Design review of the part built by this model. Coordinates are the model's own, in mm. A direction names the side the tool comes from. Give positions to 0.01 mm unless a question says otherwise; leave off trailing zeros. Loops run counter-clockwise (first coordinate to the right, second up) from the corner with the lowest first, then second, coordinate; pieces in that order, holes last.
Autodesk Fusion 360 part; units mm, degrees
sketch "Sketch1" plane through (0, 0, 0) normal (0, 0, 1) x (1, 0, 0)
  line L0 (0, 0) -> (-30, 0)
  line L1 (-30, 0) -> (-30, 30)
  line L2 (-30, 30) -> (0, 30)
  line L3 (0, 30) -> (0, 0)
  dimension "d1" = 30
  dimension "d2" = 30
extrude "Extrude1" add sketch "Sketch1" along normal blind 30
sketch "Sketch2" plane through (0, 0, 30) normal (0, 0, 1) x (-1, 0, 0)
  line L0 (0, -30) -> (30, -30)
  line L1 (30, -30) -> (30, 0)
  line L2 (30, 0) -> (0, 0)
  line L3 (0, 0) -> (0, -30)
  line L4 (30, 0) -> (25.5, 0)
  line L5 (25.5, 0) -> (25.5, -2)
  line L6 (25.5, -2) -> (30, -2)
  line L7 (30, -2) -> (30, 0)
  line L8 (25.5, -2) -> (4.5, -2)
  line L9 (4.5, -2) -> (4.5, -9)
  line L10 (4.5, -9) -> (25.5, -9)
  line L11 (25.5, -9) -> (25.5, -2)
  dimension "d5" = 4.5
  dimension "d6" = 2
  dimension "d7" = 21
  dimension "d8" = 7
extrude "Extrude2" cut sketch "Sketch2" against normal blind 25 contours L8 L9 L10 L11
sketch "Sketch3" plane through (0, 0, 0) normal (0, -1, 0) x (1, 0, 0)
  line L0 (-30, 0) -> (0, 0)
  line L1 (0, 0) -> (0, 30)
  line L2 (0, 30) -> (-30, 30)
  line L3 (-30, 30) -> (-30, 0)
  line L4 (-6, 6) -> (-24, 6)
  line L5 (-24, 6) -> (-24, 24)
  line L6 (-24, 24) -> (-6, 24)
  line L7 (-6, 24) -> (-6, 6)
  line L8 (-6, 6) -> (-24, 24) construction
  line L9 (-24, 6) -> (-6, 24) construction
  point P0 (-15, 15)
  dimension "d11" = 18
  dimension "d12" = 18
extrude "Extrude3" cut sketch "Sketch3" against normal blind 2 contours L4 L5 L6 L7
sketch "Sketch4" plane through (0, 0, 0) normal (1, 0, 0) x (0, 1, 0)
  line L0 (0, 0) -> (30, 0)
  line L1 (30, 0) -> (30, 30)
  line L2 (30, 30) -> (0, 30)
  line L3 (0, 30) -> (0, 0)
  line L4 (0, 0) -> (2, 0)
  line L5 (2, 0) -> (2, 30)
  line L6 (2, 30) -> (0, 30)
  line L7 (0, 30) -> (0, 0)
  dimension "d15" = 2
  dimension "d16" = 30
extrude "Extrude4" add sketch "Sketch4" along normal blind 2 contours L0 L2 L3 L4 L5 L6 L7
sketch "Sketch5" plane through (-30, 0, 0) normal (-1, 0, 0) x (0, -1, 0)
  line L0 (-30, 0) -> (0, 0)
  line L1 (0, 0) -> (0, 30)
  line L2 (0, 30) -> (-30, 30)
  line L3 (-30, 30) -> (-30, 0)
  line L4 (0, 0) -> (-2, 0)
  line L5 (-2, 0) -> (-2, 30)
  line L6 (-2, 30) -> (0, 30)
  line L7 (0, 30) -> (0, 0)
  dimension "d19" = 2
  dimension "d20" = 30
extrude "Extrude5" add sketch "Sketch5" along normal blind 2 contours L0 L1 L2 L4 L5 L6 L7
sketch "Sketch6" plane through (0, 0, 5) normal (0, 0, 1) x (-1, 0, 0)
  line L0 (25.5, -9) -> (25.5, -2)
  line L1 (25.5, -2) -> (4.5, -2)
  line L2 (4.5, -2) -> (4.5, -9)
  line L3 (4.5, -9) -> (25.5, -9)
  circle A0 centre (6, -5) radius 1
  dimension "d23" = 2
extrude "Extrude6" cut sketch "Sketch6" against normal blind 5 contours A0
sketch "Sketch7" plane through (0, 0, 0) normal (0, -1, 0) x (1, 0, 0)
  line L0 (-24, 6) -> (-24, 24)
  line L1 (-24, 24) -> (-6, 24)
  line L2 (-6, 24) -> (-6, 6)
  line L3 (-6, 6) -> (-24, 6)
  line L4 (-32, 0) -> (2, 0)
  line L5 (2, 0) -> (2, 30)
  line L6 (2, 30) -> (-32, 30)
  line L7 (-32, 30) -> (-32, 0)
  line L8 (-6, 6) -> (-24, 6)
  line L9 (-24, 6) -> (-24, 24)
  line L10 (-24, 24) -> (-6, 24)
  line L11 (-6, 24) -> (-6, 6)
extrude "Extrude7" cut sketch "Sketch7" against normal blind 28 contours L0 L1 L2 L3 L8 L9 L10 L11
fillet "Fillet1" radius 10 1 edges at (-15, 30, 30)
sketch "Sketch8" plane through (0, 0, 6) normal (0, 0, 1) x (-1, 0, 0)
  line L0 (24, -9) -> (6, -9)
  line L1 (6, -9) -> (6, -28)
  line L2 (6, -28) -> (24, -28)
  line L3 (24, -28) -> (24, -9)
  line L4 (24, -28) -> (6, -28)
  line L5 (6, -28) -> (6, -9)
  line L6 (6, -9) -> (24, -9)
  line L7 (24, -9) -> (24, -28)
sketch "Sketch9" plane through (0, 0, 6) normal (0, 0, 1) x (-1, 0, 0)
  line L0 (6, -9) -> (8, -9)
  line L1 (8, -9) -> (8, -11)
  line L2 (8, -11) -> (6, -11)
  line L3 (6, -11) -> (6, -9)
  line L4 (6, -11) -> (24, -11)
  line L5 (24, -11) -> (24, -28)
  line L6 (24, -28) -> (6, -28)
  line L7 (6, -28) -> (6, -11)
  point P0 (6, -9)
  point P1 (24, -28)
  dimension "d30" = 2
  dimension "d31" = 2
extrude "Extrude8" cut sketch "Sketch9" against normal blind 10 contours L2 L4 L5 L6 L7
extrude "Extrude9" cut 1 faces at (-29.3333, 0, 18) along direction (0, 1, 0) blind 0.2
sketch "Sketch10" plane through (0, 0, 0) normal (0, 0, -1) x (1, 0, 0)
  line L0 (2, -0.2) -> (-32, -0.2)
  line L1 (-32, -0.2) -> (-32, -2)
  line L2 (-32, -2) -> (-30, -2)
  line L3 (-30, -2) -> (-30, -30)
  line L4 (-30, -30) -> (0, -30)
  line L5 (0, -30) -> (0, -2)
  line L6 (0, -2) -> (2, -2)
  line L7 (2, -2) -> (2, -0.2)
  circle A0 centre (-6, -5) radius 1
  line L8 (-24, -28) -> (-24, -11)
  line L9 (-24, -11) -> (-6, -11)
  line L10 (-6, -11) -> (-6, -28)
  line L11 (-6, -28) -> (-24, -28)
extrude "Extrude10" add sketch "Sketch10" against normal blind 5 contours A0
extrude "Extrude11" cut 1 faces at (-11.5, 6.6667, 5) along direction (0, 0, -1) blind 1
sketch "Sketch11" plane through (0, 0, 4) normal (0, 0, 1) x (-1, 0, 0)
  line L0 (25.5, -9) -> (25.5, -2)
  line L1 (25.5, -2) -> (4.5, -2)
  line L2 (4.5, -2) -> (4.5, -9)
  line L3 (4.5, -9) -> (25.5, -9)
  circle A0 centre (8.1497, -5.5) radius 2
  dimension "d40" = 4
extrude "Extrude12" cut sketch "Sketch11" against normal blind 4 contours A0
extrude "Extrude13" cut 1 faces at (2, 0.8, 20) along direction (-1, 0, 0) blind 0.2
extrude "Extrude14" cut 1 faces at (-32, 1.4, 20) along direction (1, 0, 0) blind 0.2
extrude "Extrude15" cut 1 faces at (1.8, 0.8, 20) along direction (-1, 0, 0) blind 0.1
extrude "Extrude16" cut 1 faces at (-29.2, 0.2, 18) along direction (0, 1, 0) blind 0.2
extrude "Extrude17" cut 1 faces at (-31.8, 1.4667, 20) along direction (1, 0, 0) blind 0.1
Q1. Insertion check: pin 1 (5 mm diameter, centred on y = 8.5, z = 16, fed in from -X); pin 2 (2 mm diameter, centred on x = -8, z = 24.5, fed in from +Y); pin 3 (8 mm diameter, centred on x = -19.5, y = 23.5, fed in from -Z); pin 4 (3.5 mm diameter, centred on x = -8.15, y = 5.5, fed in from -Z). Each pin has a flat end and moves straight along its axis. Give the tip position at first contact, or say it passes through.
Results:
pin 1: stops at x = -30
pin 2: stops at y = 29.37
pin 3: stops at z = 24
pin 4: passes through
Q2. Take a section at A-A (y = 5.5). Give the boundary of the cut face in (x, z), plus the area to 3 significant figures.
Results:
outline: (-30, 0) - (-10.15, 0) - (-10.15, 4) - (-25.5, 4) - (-25.5, 30) - (-30, 30) - close; (-6.15, 0) - (0, 0) - (0, 30) - (-4.5, 30) - (-4.5, 4) - (-6.15, 4) - close
area: 338 mm2
Q3. Take a section at B-B (z = 3.25). Give the boundary of the cut face in (x, y), plus the area to 3 significant figures.
Results:
outline: (-31.7, 0.4) - (1.7, 0.4) - (1.7, 2) - (0, 2) - (0, 30) - (-30, 30) - (-30, 2) - (-31.7, 2) - close; hole (-24, 11) - (-6, 11) - (-6, 28) - (-24, 28) - close; hole circle Ø4 at (-8.15, 5.5)
area: 575 mm2
Q4. Take a section at D-D (y = 18.25). Give the boundary of the cut face in (x, z), plus the area to 3 significant figures.
Results:
outline: (-30, 0) - (-24, 0) - (-24, 24) - (-6, 24) - (-6, 0) - (0, 0) - (0, 30) - (-30, 30) - close
area: 468 mm2
Q5. Tool access review of faces 4 (the face through (-25.5, 6, 17)), 5 (the face through (-15, 11, 3)), 6 (the face through (-15, 10, 6)): name each direction out of +Z, -Z, +X, -X, +Y, -Y from which nothing blocks a thin tool from reaching the whole face with its end or side.
Results:
face 4: +Z
face 5: -Z
face 6: -Y
Q6. Draft analysis for pull direction X (two halves, no side actions). For faces 1 (the face through (-9.997, 6.266, 2.028)), 2 (the face through (1, 2, 15)), 3 (the face through (0, 16, 15)), state which applies: pulls with the +X half, pulls with the -X half, needs draft (parallel to the pull), parting line crosses it, or undercut.
Results:
face 1: undercut
face 2: needs draft
face 3: pulls with the +X half
Q7. Wall thickness on line 1 (X direction, y = 22, z = 9.5); line 2 (Y direction, x = -5, z = 7); line 3 (X direction, y = 5.5, z = 1.5): over which ranges is each line inside the solid? List them lowest first.
Results:
line 1: x = -30 to -24, -6 to 0
line 2: y = 0.4 to 2, 9 to 30
line 3: x = -30 to -10.15, -6.15 to 0
Q8. Take a section at C-C (x = -20.5). Give the boundary of the cut face in (y, z).
Results:
outline: (0.4, 0) - (11, 0) - (11, 6) - (9, 6) - (9, 4) - (2, 4) - (2, 6) - (0.4, 6) - close; (0.4, 24) - (2, 24) - (2, 30) - (0.4, 30) - close; (9, 24) - (28, 24) - (28, 0) - (30, 0) - (30, 20) arc R10 ccw to (20, 30) - (9, 30) - close
